```python
from build123d import *

# Parameters (mm, degrees)
BOSS_EXTRUDE1_DEPTH = 100
CUT_EXTRUDE1_DEPTH  = 102.78182549
LPATTERN1_COUNT     = 3
LPATTERN1_PITCH     = 35


with BuildPart() as part:
    # Sketch1 → Boss-Extrude1 (new body)
    with BuildSketch(Plane(origin=(0, 0, 0), x_dir=(0, 0, -1), z_dir=(1, 0, 0))):
        with BuildLine():
            Line((-6.5, 17.5), (-7.1, 17.5))
            ThreePointArc((-7.1, 17.5), (-7.241421356, 17.441421356), (-7.3, 17.3))
            Line((-7.3, 17.3), (-7.3, 13.5))
            ThreePointArc((-7.3, 13.5), (-6.860660172, 12.439339828), (-5.8, 12))
            Line((-5.8, 12), (-3, 12))
            ThreePointArc((-3, 12), (-1.939339828, 11.560660172), (-1.5, 10.5))
            Line((-1.5, 10.5), (-1.5, -10.5))
            ThreePointArc((-1.5, -10.5), (-1.939339828, -11.560660172), (-3, -12))
            Line((-3, -12), (-5.8, -12))
            ThreePointArc((-5.8, -12), (-6.860660172, -12.439339828), (-7.3, -13.5))
            Line((-7.3, -13.5), (-7.3, -17.3))
            ThreePointArc((-7.3, -17.3), (-7.241421356, -17.441421356), (-7.1, -17.5))
            Line((-7.1, -17.5), (-6.5, -17.5))
            ThreePointArc((-6.5, -17.5), (-6.358578644, -17.441421356), (-6.3, -17.3))
            Line((-6.3, -17.3), (-6.3, -15.462610506))
            Line((-6.3, -15.462610506), (-5.3, -13.5))
            Line((-5.3, -13.5), (-1.5, -13.5))
            ThreePointArc((-1.5, -13.5), (-0.439339828, -13.060660172), (0, -12))
            Line((0, -12), (0, 12))
            ThreePointArc((0, 12), (-0.439339828, 13.060660172), (-1.5, 13.5))
            Line((-1.5, 13.5), (-5.3, 13.5))
            Line((-5.3, 13.5), (-6.3, 15.462610506))
            Line((-6.3, 15.462610506), (-6.3, 17.3))
            ThreePointArc((-6.3, 17.3), (-6.358578644, 17.441421356), (-6.5, 17.5))
        make_face()
    extrude(amount=BOSS_EXTRUDE1_DEPTH)

    # Sketch2 → Cut-Extrude1 (cut, through all)
    with BuildSketch(Plane.XY):
        with BuildLine():
            Line((62.25, 2.25), (82.75, 2.25))
            ThreePointArc((82.75, 2.25), (85, 0), (82.75, -2.25))
            Line((82.75, -2.25), (62.25, -2.25))
            ThreePointArc((62.25, -2.25), (60, 0), (62.25, 2.25))
        make_face()
    cut_extrude1 = extrude(amount=CUT_EXTRUDE1_DEPTH, mode=Mode.SUBTRACT)

    # LPattern1: Cut-Extrude1 ×3
    with Locations(*[(-i * LPATTERN1_PITCH, 0, 0) for i in range(1, LPATTERN1_COUNT)]):
        add(cut_extrude1, mode=Mode.SUBTRACT)


solid = part.part
```
Model file for the job. Use its own axes, mm. A direction names the side the tool comes from. Give positions to 0.01 mm unless a question says otherwise; leave off trailing zeros. Write each loop counter-clockwise with the first axis right and the second up, starting at its lowest first coordinate (ties: lowest second). Pieces come first, ordered by that corner, then holes. Notation, with made-up numbers: M 61,44.25 L 75,44.25 A5 ccw 75,51.25 Z; hole C 77.5,17 d6. An arc over 180 degrees is marked long. Use a Markdown table: item, result.
1) Pull direction Y, two halves, no side cores. Call faces 1 (the flat face through (0, 12.2, 2.9)), 2 (the flat face through (49.3, 2.5, 1.5)), 3 (the flat face through (49, -13.5, 3)): +Y half, -Y half, draft (parallel to the pull), parting line (faces both ways), or undercut.
Responses:
| item | result |
|---|---|
| face 1 | draft |
| face 2 | undercut |
| face 3 | -Y half |
2) Cut at D-D (y = 7). List the corners of the cut face in (x, z), and give its area (3 significant figures).
Responses:
| item | result |
|---|---|
| outline | M 0,0 L 100,0 L 100,1.5 L 0,1.5 Z |
| area | 150 mm2 |
3) Cut at A-A (x = 70). List the corners of the cut face in (y, z).
Responses:
| item | result |
|---|---|
| outline | M -17.5,6.5 A0.2 ccw -17.3,6.3 L -15.46,6.3 L -13.5,5.3 L -13.5,1.5 A1.5 ccw -12,0 L -2.25,0 L -2.25,1.5 L -10.5,1.5 A1.5 cw -12,3 L -12,5.8 A1.5 ccw -13.5,7.3 L -17.3,7.3 A0.2 ccw -17.5,7.1 Z; M 2.25,0 L 12,0 A1.5 ccw 13.5,1.5 L 13.5,5.3 L 15.46,6.3 L 17.3,6.3 A0.2 ccw 17.5,6.5 L 17.5,7.1 A0.2 ccw 17.3,7.3 L 13.5,7.3 A1.5 ccw 12,5.8 L 12,3 A1.5 cw 10.5,1.5 L 2.25,1.5 Z |
4) Drill centre lines: line 1 (X direction, y = 0, z = 1); line 2 (Y direction, x = 36.5, z = 3.5); line 3 (X direction, y = -1.5, z = 0.5). Where is each one in solid material? Low to high. Write a range as from..to.
Responses:
| item | result |
|---|---|
| line 1 | x = 15..25, 50..60, 85..100 |
| line 2 | y = -13.5..-12, 12..13.5 |
| line 3 | x = 14.43..25.57, 49.43..60.57, 84.43..100 |
5) Tool access for faces 4 (the flat face through (49, -16, 6.3)), 5 (the flat face through (49, -12, 4)), 6 (the flat face through (49, 16, 6.3)), 7 (the cylindrical face through (85, 0, 1)): list every direction of +Z, -Z, +X, -X, +Y, -Y with a clear straight run to the whole face (end or side of a thin tool).
Responses:
| item | result |
|---|---|
| face 4 | -Z, +X, -X, -Y |
| face 5 | +Z, +X, -X |
| face 6 | -Z, +X, -X, +Y |
| face 7 | +Z, -Z |
6) Cut at B-B (y = 0). List the corners of the cut face in (x, z), and give its area (3 significant figures).
Responses:
| item | result |
|---|---|
| outline | M 15,0 L 25,0 L 25,1.5 L 15,1.5 Z; M 50,0 L 60,0 L 60,1.5 L 50,1.5 Z; M 85,0 L 100,0 L 100,1.5 L 85,1.5 Z |
| area | 52.5 mm2 |
7) Pin check, flat tips, straight feed: pin 1 (1 mm diameter, centred on x = 52.5, z = 1.5, fed in from -Y); pin 2 (2 mm diameter, centred on x = 31.5, z = 4.5, fed in from +Y); pin 3 (0.9 mm diameter, centred on x = 52, y = 16, fed in from -Z); pin 4 (4 mm diameter, centred on y = 9.5, z = 4, fed in from +X). Stop position of each tip, or through.
Responses:
| item | result |
|---|---|
| pin 1 | stops at y = -13.5 |
| pin 2 | stops at y = 13.89 |
| pin 3 | stops at z = 6.3 |
| pin 4 | passes through |
8) Cut at C-C (x = 93). List the corners of the cut face in (y, z).
Responses:
| item | result |
|---|---|
| outline | M -17.5,6.5 A0.2 ccw -17.3,6.3 L -15.46,6.3 L -13.5,5.3 L -13.5,1.5 A1.5 ccw -12,0 L 12,0 A1.5 ccw 13.5,1.5 L 13.5,5.3 L 15.46,6.3 L 17.3,6.3 A0.2 ccw 17.5,6.5 L 17.5,7.1 A0.2 ccw 17.3,7.3 L 13.5,7.3 A1.5 ccw 12,5.8 L 12,3 A1.5 cw 10.5,1.5 L -10.5,1.5 A1.5 cw -12,3 L -12,5.8 A1.5 ccw -13.5,7.3 L -17.3,7.3 A0.2 ccw -17.5,7.1 Z |
